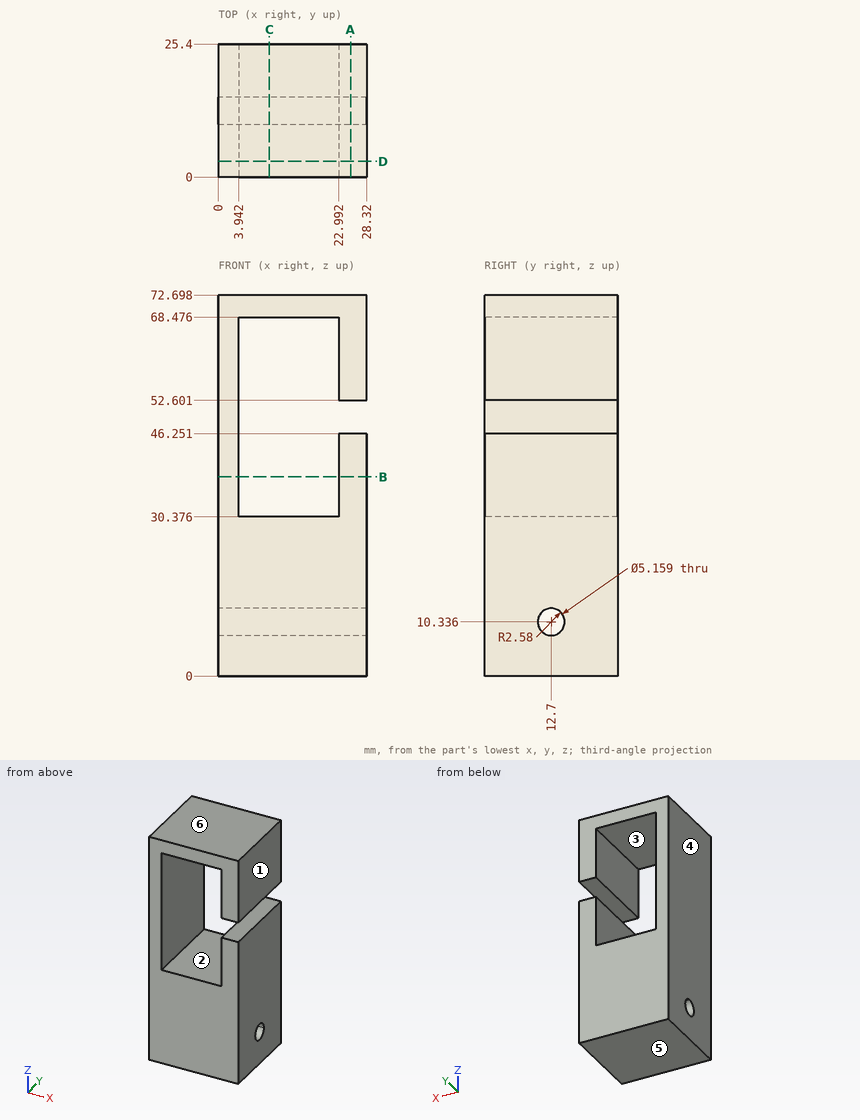
Verification items for this drawing (mm, ordinates from the low corner). A direction names the side the tool comes from. Coordinates: 2 decimals unless noted, no trailing zeros. Loops run counter-clockwise (first coordinate to the right, second up) from the corner with the lowest first, then second, coordinate; pieces in that order, holes last. Notation, with made-up numbers: (43, 33) -> (67, 33) arc R16 cw to (67, 39) -> close; hole circle Ø6 at (22.5, -30). An arc over 180 degrees is marked (long way). Put each result on its own line as item: value.
1. Thickness scan on line 1 (Z direction, x = 19.75, y = 12.7) (1 decimal); line 2 (X direction, y = 23.5, z = 56.5); line 3 (Z direction, x = 13.25, y = 15.5). Record the ranges inside material, lowest first.
Result set:
line 1: z = 0 to 7.8, 12.9 to 30.4, 68.5 to 72.7
line 2: x = 0 to 3.94, 22.99 to 28.32
line 3: z = 0 to 30.38, 68.48 to 72.7
2. Tool access check on the marked faces 1 and 2. Record the directions out of +Z, -Z, +X, -X, +Y, -Y that give a thin tool (end or side, any length) a straight path to the whole face; none if there is none.
Result set:
face 1: +Z, -Z, +X, +Y, -Y
face 2: +Y, -Y
3. Gauge pin test, flat end, axial feed: P1, Ø4.5, axis at y = 12.7, z = 10.34, coming from the -X side. Record the tip position at first contact, or that the pin passes through.
Result set:
P1: passes through
4. Mould release check, pull along Z, two halves, no side actions. Record for the marked faces 3, 4, 5 and 6: pulls with the +Z half, pulls with the -Z half, needs draft (parallel to the pull), parting line crosses it, or undercut.
Result set:
face 3: undercut
face 4: needs draft
face 5: pulls with the -Z half
face 6: pulls with the +Z half
5. Section check C-C, the plane x = 9.75. Record the boundary of the cut face in (y, z) (1 decimal).
Result set:
outline: (0, 0) -> (25.4, 0) -> (25.4, 30.4) -> (0, 30.4) -> close; (0, 68.5) -> (25.4, 68.5) -> (25.4, 72.7) -> (0, 72.7) -> close; hole circle Ø5.2 at (12.7, 10.3)
6. Section check A-A, the plane x = 25.25. Record the boundary of the cut face in (y, z) (1 decimal).
Result set:
outline: (0, 0) -> (25.4, 0) -> (25.4, 46.3) -> (0, 46.3) -> close; (0, 52.6) -> (25.4, 52.6) -> (25.4, 72.7) -> (0, 72.7) -> close; hole circle Ø5.2 at (12.7, 10.3)
7. Section check B-B, the plane z = 38. Record the boundary of the cut face in (x, y).
Result set:
outline: (0, 0) -> (3.94, 0) -> (3.94, 25.4) -> (0, 25.4) -> close; (22.99, 0) -> (28.32, 0) -> (28.32, 25.4) -> (22.99, 25.4) -> close
8. Section check D-D, the plane y = 3. Record the boundary of the cut face in (x, z), then the cut area to 3 significant figures.
Result set:
outline: (0, 0) -> (28.32, 0) -> (28.32, 46.25) -> (22.99, 46.25) -> (22.99, 30.38) -> (3.94, 30.38) -> (3.94, 68.48) -> (22.99, 68.48) -> (22.99, 52.6) -> (28.32, 52.6) -> (28.32, 72.7) -> (0, 72.7) -> close
area: 1,300 mm^2
